The figure shows three views and two pictorial views of one solid part (mm, origin at its lowest corner). Answer the questions. A direction names the side the tool comes from. Round coordinates to 2 decimals unless told otherwise and drop trailing zeros. Order: outer loops, then holes, each group sorted by start corner. A loop starts at its lowest first (then second) coordinate and runs counter-clockwise, first axis right, second up. Notation, with made-up numbers: (38.5, 51.25) -> (89.5, 51.25) arc R17 cw to (89.5, 65.25) -> close; hole circle Ø1 at (-35, 89). An arc over 180 degrees is marked (long way). Return JSON: item names as keys, results as strings. Group by question number.
(1) Consider line 1 (Y direction, x = 25, z = 0.7); line 2 (Y direction, x = 44, z = 28.5). Determine where each line is inside the solid, lowest interval first. Write a range as [from, to].
(2) The part is cut by section C-C (y = 28). Determine the outline of the cut face in (x, z).
(3) Each of these flat-tipped pins is pushed along its axis until it touches: pin 1 (4 mm diameter, centred on x = 39.5, y = 28, fed in from -Z); pin 2 (25 mm diameter, centred on x = 25.5, z = 20.5, fed in from +Y); pin 3 (1 mm diameter, centred on x = 27, y = 18.5, fed in from +Z). Where does it stop, or does it pass through?
(4) The part is cut by section D-D (x = 43). Determine the outline of the cut face in (y, z).
(5) The part is cut by section B-B (x = 25). Determine the outline of the cut face in (y, z).
(6) The part is cut by section A-A (z = 11). Determine the outline of the cut face in (x, y).
(7) Which of the six approach directions +Z, -Z, +X, -X, +Y, -Y give full straight-line access (tool end or side, diameter ignored) to the marked faces 1 and 2?
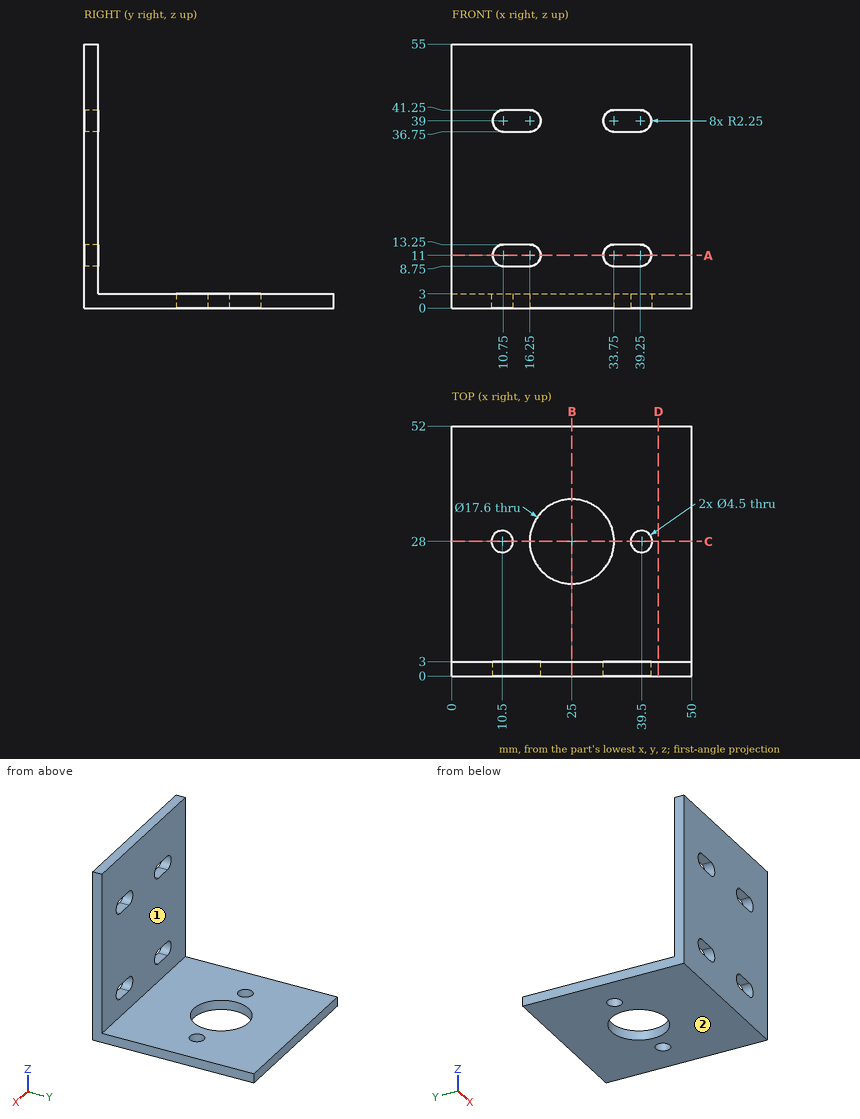
Answer below:
{
 "1": {"line 1": "y = [0, 19.2], [36.8, 52]", "line 2": "y = [0, 3]"},
 "2": {"outline": "(0, 0) -> (8.25, 0) -> (8.25, 3) -> (0, 3) -> close; (12.75, 0) -> (16.2, 0) -> (16.2, 3) -> (12.75, 3) -> close; (33.8, 0) -> (37.25, 0) -> (37.25, 3) -> (33.8, 3) -> close; (41.75, 0) -> (50, 0) -> (50, 3) -> (41.75, 3) -> close"},
 "3": {"pin 1": "passes through", "pin 2": "stops at y = 3", "pin 3": "stops at z = 3"},
 "4": {"outline": "(0, 0) -> (52, 0) -> (52, 3) -> (3, 3) -> (3, 55) -> (0, 55) -> close"},
 "5": {"outline": "(0, 0) -> (19.2, 0) -> (19.2, 3) -> (3, 3) -> (3, 55) -> (0, 55) -> close; (36.8, 0) -> (52, 0) -> (52, 3) -> (36.8, 3) -> close"},
 "6": {"outline": "(0, 0) -> (8.5, 0) -> (8.5, 3) -> (0, 3) -> close; (18.5, 0) -> (31.5, 0) -> (31.5, 3) -> (18.5, 3) -> close; (41.5, 0) -> (50, 0) -> (50, 3) -> (41.5, 3) -> close"},
 "7": {"face 1": "+Z, +X, -X, +Y", "face 2": "-Z, +X, -X, +Y, -Y"}
}
